Verification items for this drawing (mm, ordinates from the low corner). A direction names the side the tool comes from. Give positions to 0.01 mm unless a question says otherwise; leave off trailing zeros. Order: outer loops, then holes, each group sorted by start corner. A loop starts at its lowest first (then second) coordinate and runs counter-clockwise, first axis right, second up. Notation, with made-up numbers: M 13,51 L 36,51 A5 cw 36,55 Z; hole C 29.5,28.5 d9. An arc over 180 degrees is marked long. Return JSON: item names as keys, results as strings. Group by question number.
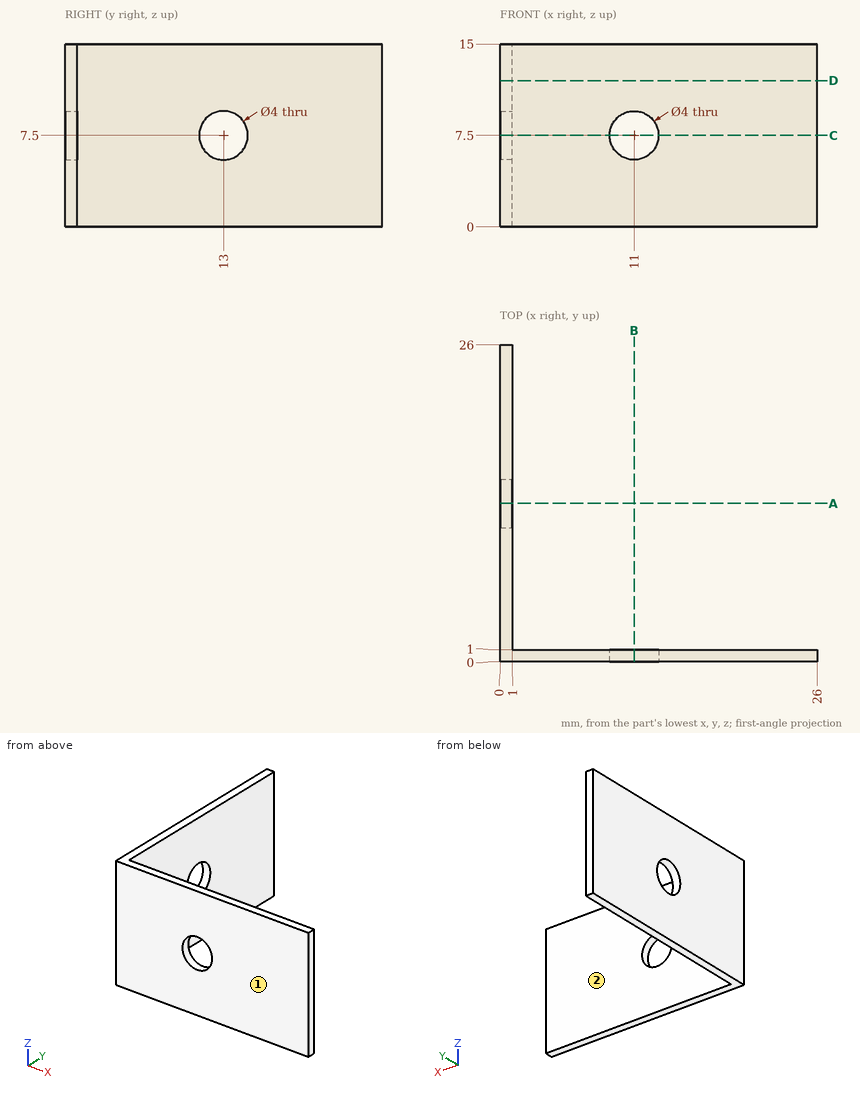
1) Sectioned sample at A-A on y = 13. Record the boundary of the cut face in (x, z).
2) Tool access check on the marked faces 1 and 2. Record the directions out of +Z, -Z, +X, -X, +Y, -Y that give a thin tool (end or side, any length) a straight path to the whole face; none if there is none.
3) Sectioned sample at C-C on z = 7.5. Record the boundary of the cut face in (x, y), then the cut area to 3 significant figures.
4) Material ranges on line 1 along X through (y, z) = (0.6, 7.5); line 2 along Z through (x, y) = (11, 0.55); line 3 along Y through (x, z) = (0.25, 7.5), recorded low to high.
5) Sectioned sample at D-D on z = 12. Record the boundary of the cut face in (x, y).
6) Depth check by flat-ended pin: P1, Ø1.5, axis at y = 10.5, z = 3.5, coming from the +X side; P2, Ø7.5, axis at x = 7.5, z = 5, coming from the +Y side. Enter the tip coordinate at first touch or a pass-through.
Reply:
{
 "1": {"outline": "M 0,0 L 1,0 L 1,5.5 L 0,5.5 Z; M 0,9.5 L 1,9.5 L 1,15 L 0,15 Z"},
 "2": {"face 1": "+Z, -Z, +X, -X, -Y", "face 2": "+Z, -Z, +X, +Y"},
 "3": {"outline": "M 0,0 L 9,0 L 9,1 L 1,1 L 1,11 L 0,11 Z; M 0,15 L 1,15 L 1,26 L 0,26 Z; M 13,0 L 26,0 L 26,1 L 13,1 Z", "area": "43.0 mm^2"},
 "4": {"line 1": "0 to 9, 13 to 26", "line 2": "0 to 5.5, 9.5 to 15", "line 3": "0 to 11, 15 to 26"},
 "5": {"outline": "M 0,0 L 26,0 L 26,1 L 1,1 L 1,26 L 0,26 Z"},
 "6": {"P1": "x = 1", "P2": "y = 1"}
}
